Source: CAD feature listing. Evaluate the final solid. Frame: model axes, mm. A direction names the side the tool comes from. Give positions to 0.01 mm unless a question says otherwise; leave off trailing zeros. Order: outer loops, then holes, each group sorted by start corner. A loop starts at its lowest first (then second) coordinate and runs counter-clockwise, first axis right, second up. Notation, with made-up numbers: M -2.75,64 L 28.25,64 A19 ccw 28.25,70 Z; hole C 37,-30 d9. An arc over 180 degrees is marked long. Answer in a Markdown table with one row per item. Add a question column.
(1) Mould query, pull axis Y, two halves, no side actions, for faces 1 (the face through (-23.25, -38.4, 14.7)), 2 (the face through (0, -29.5, 29)), 3 (the face through (23.19, 38.35, 14.7)). Classes: pulls with the +Y half, pulls with the -Y half, needs draft (parallel to the pull), parting line crosses it, or undercut.
(2) Section query B-B, the plane z = 4. Return loops of the section in (x, y).
(3) Material intervals for line 1 along Y through (x, z) = (-16, 2.5); line 2 along X through (y, z) = (-7, 18); line 3 along Y through (x, z) = (-23, 22), sorted ascending.
(4) Pin query (flat end, axial travel): P1, Ø0.5, axis at x = -22.5, y = 33, coming from the -Z side; P2, Ø0.6, axis at x = -0.5, z = 29, coming from the -Y side; P3, Ø8.5, axis at x = -1, z = 9, coming from the +Y side. Return the tip coordinate at first contact, or that it passes through.
(5) Section query D-D, the plane x = -12. Return loops of the section in (y, z).
(6) Set-up query: faces 4 (the face through (-23, -30.7, 17)), 5 (the face through (7, -24.5, 29)), 6 (the face through (28.4, 33.25, 14.7)), 7 (the face through (0, 37.5, 14)). Return all of +Z, -Z, +X, -X, +Y, -Y with unobstructed straight access to the full face (end or side cutting, diameter ignored); none if empty.
(7) Section query C-C, the plane y = -12. Return loops of the section in (x, z).
(8) Section query A-A, the plane y = 3. Return loops of the section in (x, z).
from build123d import *

# Parameters (mm, degrees)
SKETCH_R        = 1.5
PAD_DEPTH       = 30
SKETCH001_W     = 51
SKETCH001_H     = 71
POCKET_DEPTH    = 28
SKETCH002_W     = 4.8
SKETCH002_H     = 4.8
SKETCH002_R     = 0.9
PAD001_DEPTH    = 23
SKETCH003_W     = 4.8
SKETCH003_H     = 4.8
SKETCH003_R     = 0.9
PAD002_DEPTH    = 23
SKETCH004_W     = 4.8
SKETCH004_H     = 4.8
SKETCH004_R     = 0.9
PAD003_DEPTH    = 23
SKETCH005_W     = 4.8
SKETCH005_H     = 4.8
SKETCH005_R     = 0.9
PAD004_DEPTH    = 23
SKETCH006_R     = 5
POCKET001_DEPTH = 5
SKETCH007_R     = 8
POCKET002_DEPTH = 5
POCKET003_DEPTH = 5
SKETCH009_W     = 13
SKETCH009_H     = 10
POCKET004_DEPTH = 5
SKETCH010_R     = 0.75
POCKET005_DEPTH = 5
FILLET002_R     = 4
FILLET003_R     = 1


with BuildPart() as part:
    # Sketch → Pad (new body)
    with BuildSketch(Plane.XY):
        with BuildLine():
            ThreePointArc((-24.917424, 37.5), (-33.035534, 43.035534), (-27.5, 34.917424))
            Line((-27.5, 34.917424), (-27.5, -34.917424))
            ThreePointArc((-27.5, -34.917424), (-33.035534, -43.035534), (-24.917424, -37.5))
            Line((-24.917424, -37.5), (24.917424, -37.5))
            ThreePointArc((24.917424, -37.5), (33.035534, -43.035534), (27.5, -34.917424))
            Line((27.5, 34.917424), (27.5, -34.917424))
            ThreePointArc((27.5, 34.917424), (33.035534, 43.035534), (24.917424, 37.5))
            Line((-24.917424, 37.5), (24.917424, 37.5))
        make_face()
        with Locations((-29.5, 39.5)):
            Circle(SKETCH_R, mode=Mode.SUBTRACT)
        with Locations((29.5, 39.5)):
            Circle(SKETCH_R, mode=Mode.SUBTRACT)
        with Locations((-29.5, -39.5)):
            Circle(SKETCH_R, mode=Mode.SUBTRACT)
        with Locations((29.5, -39.5)):
            Circle(SKETCH_R, mode=Mode.SUBTRACT)
    extrude(amount=PAD_DEPTH)

    # Sketch001 (on Face13 of Pad) → Pocket (cut)
    with BuildSketch(Plane(origin=(0, 0, 0), x_dir=(1, 0, 0), z_dir=(0, 0, -1))):
        Rectangle(SKETCH001_W, SKETCH001_H)
    extrude(amount=-POCKET_DEPTH, mode=Mode.SUBTRACT)

    # Sketch002 (on Face19 of Pocket) → Pad001 (join)
    with BuildSketch(Plane(origin=(0, 0, 28), x_dir=(1, 0, 0), z_dir=(0, 0, -1))):
        with Locations((-23.1, 33.1)):
            Rectangle(SKETCH002_W, SKETCH002_H)
        with Locations((-23, 32.9)):
            Circle(SKETCH002_R, mode=Mode.SUBTRACT)
    extrude(amount=PAD001_DEPTH)

    # Sketch003 (on Face19 of Pad001) → Pad002 (join)
    with BuildSketch(Plane(origin=(0, 0, 28), x_dir=(1, 0, 0), z_dir=(0, 0, -1))):
        with Locations((23.1, 33.1)):
            Rectangle(SKETCH003_W, SKETCH003_H)
        with Locations((23, 32.9)):
            Circle(SKETCH003_R, mode=Mode.SUBTRACT)
    extrude(amount=PAD002_DEPTH)

    # Sketch004 (on Face21 of Pad002) → Pad003 (join)
    with BuildSketch(Plane(origin=(0, 0, 28), x_dir=(1, 0, 0), z_dir=(0, 0, -1))):
        with Locations((23.1, -33.1)):
            Rectangle(SKETCH004_W, SKETCH004_H)
        with Locations((23, -32.9)):
            Circle(SKETCH004_R, mode=Mode.SUBTRACT)
    extrude(amount=PAD003_DEPTH)

    # Sketch005 (on Face21 of Pad003) → Pad004 (join)
    with BuildSketch(Plane(origin=(0, 0, 28), x_dir=(1, 0, 0), z_dir=(0, 0, -1))):
        with Locations((-23.1, -33.1)):
            Rectangle(SKETCH005_W, SKETCH005_H)
        with Locations((-23, -32.9)):
            Circle(SKETCH005_R, mode=Mode.SUBTRACT)
    extrude(amount=PAD004_DEPTH)

    # Sketch006 (on Face21 of Pad004) → Pocket001 (cut)
    with BuildSketch(Plane(origin=(0, 0, 28), x_dir=(1, 0, 0), z_dir=(0, 0, -1))):
        with Locations((0, -6)):
            Circle(SKETCH006_R)
    extrude(amount=-POCKET001_DEPTH, mode=Mode.SUBTRACT)

    # Sketch007 (on Face22 of Pocket001) → Pocket002 (cut)
    with BuildSketch(Plane(origin=(0, 0, 28), x_dir=(1, 0, 0), z_dir=(0, 0, -1))):
        with Locations((0, 12)):
            Circle(SKETCH007_R)
    extrude(amount=-POCKET002_DEPTH, mode=Mode.SUBTRACT)

    # Sketch008 (on Face23 of Pocket002) → Pocket003 (cut)
    with BuildSketch(Plane(origin=(0, 0, 28), x_dir=(1, 0, 0), z_dir=(0, 0, -1))):
        with BuildLine():
            ThreePointArc((-6, 29.5), (-7, 28.5), (-6, 27.5))
            Line((-6, 27.5), (6, 27.5))
            ThreePointArc((6, 27.5), (7, 28.5), (6, 29.5))
            Line((-6, 29.5), (6, 29.5))
        make_face()
        with BuildLine():
            ThreePointArc((-6, 25.5), (-7, 24.5), (-6, 23.5))
            Line((-6, 23.5), (6, 23.5))
            ThreePointArc((6, 23.5), (7, 24.5), (6, 25.5))
            Line((-6, 25.5), (6, 25.5))
        make_face()
    extrude(amount=-POCKET003_DEPTH, mode=Mode.SUBTRACT)

    # Sketch009 (on Face9 of Pocket003) → Pocket004 (cut)
    with BuildSketch(Plane.XZ.offset(37.5)):
        with Locations((11.5, 10.8)):
            Rectangle(SKETCH009_W, SKETCH009_H)
    extrude(amount=-POCKET004_DEPTH, mode=Mode.SUBTRACT)

    # Sketch010 (on Face37 of Pocket004) → Pocket005 (cut)
    with BuildSketch(Plane(origin=(0, 0, 28), x_dir=(1, 0, 0), z_dir=(0, 0, -1))):
        with Locations((-7.115, -26)):
            Circle(SKETCH010_R)
        with Locations((7.115, -26)):
            Circle(SKETCH010_R)
        with BuildLine():
            ThreePointArc((-2.5, -23.5), (-5, -26), (-2.5, -28.5))
            Line((-2.5, -28.5), (2.5, -28.5))
            ThreePointArc((2.5, -28.5), (5, -26), (2.5, -23.5))
            Line((-2.5, -23.5), (2.5, -23.5))
        make_face()
    extrude(amount=-POCKET005_DEPTH, mode=Mode.SUBTRACT)

    # Fillet002
    fillet002_edges = [part.edges().sort_by_distance(p)[0] for p in [
        (-27.5, 34.917424, 15),
        (-24.917424, 37.5, 15),
        (27.5, 34.917424, 15),
        (24.917424, 37.5, 15),
        (-24.917424, -37.5, 15),
        (-27.5, -34.917424, 15),
        (27.5, -34.917424, 15),
        (24.917424, -37.5, 15),
    ]]
    fillet(fillet002_edges, radius=FILLET002_R)

    # Fillet003
    fillet003_edges = [part.edges().sort_by_distance(p)[0] for p in [
        (27.5, 0, 30),
    ]]
    fillet(fillet003_edges, radius=FILLET003_R)


solid = part.part
Values follow:
| question | item | result |
|---|---|---|
| 1 | face 1 | pulls with the -Y half |
| 1 | face 2 | undercut |
| 1 | face 3 | pulls with the +Y half |
| 2 | outline | M -30.61,-34.63 A5 ccw long -24.63,-40.61 A4 cw -20.73,-37.5 L 20.73,-37.5 A4 cw 24.63,-40.61 A5 ccw long 30.61,-34.63 A4 cw 27.5,-30.73 L 27.5,30.73 A4 cw 30.61,34.63 A5 ccw long 24.63,40.61 A4 cw 20.73,37.5 L -20.73,37.5 A4 cw -24.63,40.61 A5 ccw long -30.61,34.63 A4 cw -27.5,30.73 L -27.5,-30.73 A4 cw Z; hole C -29.5,-39.5 d3; hole C -29.5,39.5 d3; hole M -25.5,-35.5 L 25.5,-35.5 L 25.5,35.5 L -25.5,35.5 Z; hole C 29.5,-39.5 d3; hole C 29.5,39.5 d3 |
| 3 | line 1 | y = -37.5 to -35.5, 35.5 to 37.5 |
| 3 | line 2 | x = -27.5 to -25.5, 25.5 to 27.5 |
| 3 | line 3 | y = -38.21 to -33.8, -32 to -30.7, 30.7 to 32, 33.8 to 38.21 |
| 4 | P1 | stops at z = 28 |
| 4 | P2 | stops at y = -37.5 |
| 4 | P3 | stops at y = 37.5 |
| 5 | outline | M -37.5,0 L -35.5,0 L -35.5,28 L 35.5,28 L 35.5,0 L 37.5,0 L 37.5,29 A1 ccw 36.5,30 L -36.5,30 A1 ccw -37.5,29 Z |
| 6 | face 4 | -Z |
| 6 | face 5 | +Z, -Z |
| 6 | face 6 | +Z, -Z, +X |
| 6 | face 7 | +Z, -Z, +Y |
| 7 | outline | M -27.5,0 L -25.5,0 L -25.5,28 L -8,28 L -8,30 L -26.5,30 A1 ccw -27.5,29 Z; M 8,28 L 25.5,28 L 25.5,0 L 27.5,0 L 27.5,29 A1 ccw 26.5,30 L 8,30 Z |
| 8 | outline | M -27.5,0 L -25.5,0 L -25.5,28 L -4,28 L -4,30 L -26.5,30 A1 ccw -27.5,29 Z; M 4,28 L 25.5,28 L 25.5,0 L 27.5,0 L 27.5,29 A1 ccw 26.5,30 L 4,30 Z |
